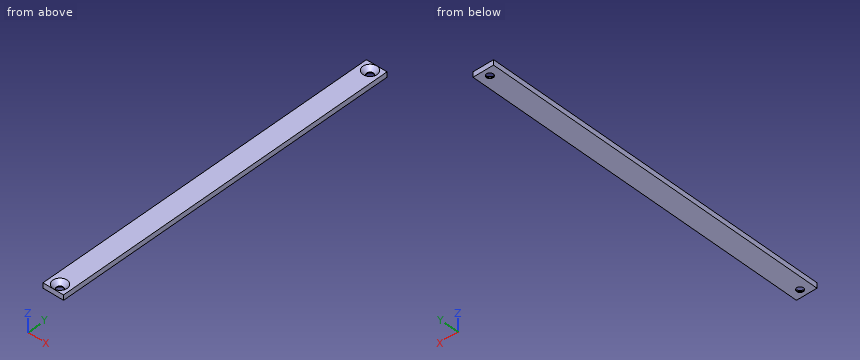
from build123d import *

# Parameters (mm, degrees)
SKETCH1_W                                    = 25.4
SKETCH1_H                                    = 431.973597558
EXTRUDE1_DEPTH                               = 6.35
CSK_FOR_5_16_FLAT_HEAD_SOCKET_CAP_SC_2_COUNT = 2
CSK_FOR_5_16_FLAT_HEAD_SOCKET_CAP_SC_2_PITCH = 414.193597559


with BuildPart() as part:
    # Sketch1 → Extrude1 (new body)
    with BuildSketch(Plane.XY):
        with Locations((-41.434947789, 0)):
            Rectangle(SKETCH1_W, SKETCH1_H)
    extrude(amount=EXTRUDE1_DEPTH)

    # Sketch4 → CSK for 5/16 Flat Head Socket Cap Screw1 (revolve, cut)
    with BuildSketch(Plane(origin=(-41.434947789, 207.096798779, 6.35), x_dir=(0, -1, 0), z_dir=(1, 0, 0))):
        Polygon((0, 0), (0, 6.35), (4.1021, 6.35), (4.1021, 5.373016172), (8.7727917, 0), align=None)
    csk_for_5_16_flat_head_socket_cap_screw1 = revolve(axis=Axis((-41.434947789, 207.096798779, 12.7), (0, 0, -1)), mode=Mode.SUBTRACT)

    # CSK for 5_16 Flat Head Socket Cap Sc 2: CSK for 5/16 Flat Head Socket Cap Screw1 ×2
    with Locations(*[(0, -i * CSK_FOR_5_16_FLAT_HEAD_SOCKET_CAP_SC_2_PITCH, 0) for i in range(1, CSK_FOR_5_16_FLAT_HEAD_SOCKET_CAP_SC_2_COUNT)]):
        add(csk_for_5_16_flat_head_socket_cap_screw1, mode=Mode.SUBTRACT)


solid = part.part
Design review of the part built by this model. Coordinates are the model's own, in mm. Give positions to 0.01 mm unless a question says otherwise; leave off trailing zeros. Loops run counter-clockwise (first coordinate to the right, second up) from the corner with the lowest first, then second, coordinate; pieces in that order, holes last. Notation, with made-up numbers: M 13.5,48.5 L 45.5,48.5 A21 cw 45.5,81.5 Z; hole C -15,71.25 d6. An arc over 180 degrees is marked long. Answer as a JSON object with one key per item and string values.
Item 1: For P1, Ø12, axis at x = -35.5, y = -132.5, coming from the -Z side; P2, Ø7.5, axis at x = -41.43, y = 207.1, coming from the +Z side, all flat-tipped, find the tip position at first contact; note any pin that passes through.
Output values:
{"P1": "stops at z = 0", "P2": "passes through"}
Item 2: We need section A-A (z = 2.5). State the section outline as (x, y) points.
Output values:
{"outline": "M -54.13,-215.99 L -28.73,-215.99 L -28.73,215.99 L -54.13,215.99 Z; hole C -41.43,-207.1 d10.85; hole C -41.43,207.1 d10.85"}
Item 3: Wall thickness on line 1 along Y through (x, z) = (-44.75, 4.25); line 2 along Y through (x, z) = (-44, 0.5): over which ranges is each line inside the solid? List them lowest first.
Output values:
{"line 1": "y = -215.99 to -213.2, -200.99 to 200.99, 213.2 to 215.99", "line 2": "y = -215.99 to -210.3, -203.9 to 203.9, 210.3 to 215.99"}
